The listing builds one solid part. Answer for the finished solid, in the listing's coordinates (mm). A direction names the side the tool comes from. Round coordinates to 2 decimals unless told otherwise and drop trailing zeros. Write each loop counter-clockwise with the first axis right and the second up, starting at its lowest first coordinate (ties: lowest second). Pieces come first, ordered by that corner, then holes. Notation, with made-up numbers: (70, 38) - (75, 38) arc R10 cw to (75, 42) - close; hole circle Ø8 at (27, 70.25). An arc over 180 degrees is marked (long way). Return JSON: item names as keys, results as strings. Group by question number.
(1) Each of these flat-tipped pins is pushed along its axis until it touches: pin 1 (2 mm diameter, centred on x = 9, z = 14, fed in from -Y); pin 2 (2 mm diameter, centred on y = -15.5, z = -15.5, fed in from -X); pin 3 (5.5 mm diameter, centred on x = -2, y = -9, fed in from +Z). Where does it stop, or does it pass through?
(2) Determine the mould class of faces 1 (the cylindrical face through (-14.316, 1.521, 19.278)), 2 (the flat face through (0, -11, -17)), 3 (the cylindrical face through (14.278, 1.521, 19.316)), 4 (the cylindrical face through (-13.67, 1.48, 8.26)) for opening direction X: +X half, -X half, draft (parallel to the pull), parting line (faces both ways), or undercut.
(3) Section D-D, the plane y = -15.75 is taken. Write down the section's boundary in (x, z), then the cut area to 3 significant figures.
(4) Which of the six approach directions +Z, -Z, +X, -X, +Y, -Y give full straight-line access (tool end or side, diameter ignored) to faces 5 (the flat face through (0, 1, 20)), 6 (the flat face through (0, 0, 2))?
(5) Section C-C, the plane x = 7.5 is taken. Write down the section's boundary in (y, z), then the cut area to 3 significant figures.
(6) Section A-A, the plane z = 8 is taken. Write down the section's boundary in (x, y), then the cut area to 3 significant figures.
(7) Find the intervals of material crossed by line 1 along X through (y, z) = (2.2, 17.5); line 2 along X through (y, z) = (1.35, 8); line 3 along Z through (x, y) = (-1.5, -6.5), in increasing order. Write a range as [from, to].
(8) Section B-B, the plane x = -5 is taken. Write down the section's boundary in (y, z).
```python
from build123d import *

# Parameters (mm, degrees)
ESBO_O1_W                = 30
ESBO_O1_H                = 40
RESSALTO_EXTRUS_O1_DEPTH = 3
ESBO_O3_R                = 1.2
CORTE_EXTRUS_O2_DEPTH    = 26.179356624
ESBO_O4_W                = 30
ESBO_O4_H                = 3
RESSALTO_EXTRUS_O2_DEPTH = 20
FILETE5_R                = 2.4
FILETE6_R                = 2.4
FILETE7_R                = 2.4
FILETE8_R                = 2.4


with BuildPart() as part:
    # Esboço1 → Ressalto-extrusão1 (new body)
    with BuildSketch(Plane(origin=(0, 0, 0), x_dir=(1, 0, 0), z_dir=(0, 1, 0))):
        Rectangle(ESBO_O1_W, ESBO_O1_H)
    extrude(amount=RESSALTO_EXTRUS_O1_DEPTH)

    # Esboço3 → Corte-extrusão2 (cut, through all)
    with BuildSketch(Plane.XZ):
        with Locations(Location((-5, 17.5, 0), (0, 0, 270))):
            Circle(ESBO_O3_R)
        with Locations(Location((-12.5, 8, 0), (0, 0, 270))):
            Circle(ESBO_O3_R)
        with Locations(Location((12.545132566, 8.047190753, 0), (0, 0, 90))):
            Circle(ESBO_O3_R)
        with Locations(Location((5.009385606, 17.51885997, 0), (0, 0, 90))):
            Circle(ESBO_O3_R)
    extrude(amount=-CORTE_EXTRUS_O2_DEPTH, mode=Mode.SUBTRACT)

    # Esboço4 → Ressalto-extrusão2 (add)
    with BuildSketch(Plane.XZ):
        with Locations((0, -18.5)):
            Rectangle(ESBO_O4_W, ESBO_O4_H)
    extrude(amount=RESSALTO_EXTRUS_O2_DEPTH)

    # Filete5
    filete5_edges = [part.edges().sort_by_distance(p)[0] for p in [
        (0, 0, -17),
    ]]
    fillet(filete5_edges, radius=FILETE5_R)

    # Filete6
    filete6_edges = [part.edges().sort_by_distance(p)[0] for p in [
        (0, 3, -20),
    ]]
    fillet(filete6_edges, radius=FILETE6_R)

    # Filete7
    filete7_edges = [part.edges().sort_by_distance(p)[0] for p in [
        (15, 1.5, 20),
        (-15, 1.5, 20),
    ]]
    fillet(filete7_edges, radius=FILETE7_R)

    # Filete8
    filete8_edges = [part.edges().sort_by_distance(p)[0] for p in [
        (-15, -20, -18.5),
        (15, -20, -18.5),
    ]]
    fillet(filete8_edges, radius=FILETE8_R)


solid = part.part
```
Working result:
{
 "1": {"pin 1": "stops at y = 0", "pin 2": "passes through", "pin 3": "stops at z = -17"},
 "2": {"face 1": "-X half", "face 2": "draft", "face 3": "+X half", "face 4": "undercut"},
 "3": {"outline": "(-15, -20) - (15, -20) - (15, -17) - (-15, -17) - close", "area": "90.0 mm^2"},
 "4": {"face 5": "+Z, +X, -X, +Y, -Y", "face 6": "+Z, +X, -X, -Y"},
 "5": {"outline": "(-20, -20) - (0.6, -20) arc R2.4 ccw to (3, -17.6) - (3, 20) - (0, 20) - (0, -14.6) arc R2.4 cw to (-2.4, -17) - (-20, -17) - close", "area": "180 mm^2"},
 "6": {"outline": "(-15, 0) - (-13.7, 0) - (-13.7, 3) - (-15, 3) - close; (-11.3, 0) - (11.35, 0) - (11.35, 3) - (-11.3, 3) - close; (13.74, 0) - (15, 0) - (15, 3) - (13.74, 3) - close", "area": "75.6 mm^2"},
 "7": {"line 1": "x = [-15, -6.2], [-3.8, 3.81], [6.21, 15]", "line 2": "x = [-15, -13.7], [-11.3, 11.35], [13.74, 15]", "line 3": "z = [-20, -17]"},
 "8": {"outline": "(-20, -20) - (0.6, -20) arc R2.4 ccw to (3, -17.6) - (3, 16.3) - (0, 16.3) - (0, -14.6) arc R2.4 cw to (-2.4, -17) - (-20, -17) - close; (0, 18.7) - (3, 18.7) - (3, 20) - (0, 20) - close"}
}
